```python
from build123d import *
from build123d.topology import SkipClean

# Parameters (mm, degrees)
ESQUISSE1_R             = 3.5
ESQUISSE1_R_2           = 8.5
BOSS_EXTRU_1_DEPTH      = 7
ESQUISSE2_R             = 23
ESQUISSE2_R_2           = 8.5
BOSS_EXTRU_2_DEPTH      = 7
ESQUISSE3_R             = 10
ESQUISSE3_R_2           = 8.5
BOSS_EXTRU_3_DEPTH      = 5.5
ENL_V_START             = -2
ESQUISSE4_R             = 21
ESQUISSE4_R_2           = 10
ENL_V_MAT_EXTRU_1_DEPTH = 2


with BuildPart() as part:
    # Esquisse1 → Boss.-Extru.1 (new body)
    with BuildSketch(Plane.XY):
        with BuildLine():
            Line((11.717444642, 19.791449948), (6, 35.5))
            ThreePointArc((6, 35.5), (0, 37.604686356), (-6, 35.5))
            Line((-6, 35.5), (-11.717444642, 19.791449948))
            ThreePointArc((-11.717444642, 19.791449948), (-23, 0), (-11.717444642, -19.791449948))
            Line((-11.717444642, -19.791449948), (-6, -35.5))
            ThreePointArc((-6, -35.5), (0, -37.604686356), (6, -35.5))
            Line((6, -35.5), (11.717444642, -19.791449948))
            ThreePointArc((11.717444642, -19.791449948), (23, 0), (11.717444642, 19.791449948))
        make_face()
        with Locations((0, 28)):
            Circle(ESQUISSE1_R, mode=Mode.SUBTRACT)
        Circle(ESQUISSE1_R_2, mode=Mode.SUBTRACT)
        with Locations(Location((0, -28, 0), (0, 0, 180))):
            Circle(ESQUISSE1_R, mode=Mode.SUBTRACT)
    extrude(amount=BOSS_EXTRU_1_DEPTH)

    # Esquisse2 → Boss.-Extru.2 (add)
    with BuildSketch(Plane.XY.offset(7)):
        with Locations(Location((0, 0, 0), (0, 0, 120.627475448))):
            Circle(ESQUISSE2_R)
        Circle(ESQUISSE2_R_2, mode=Mode.SUBTRACT)
    extrude(amount=BOSS_EXTRU_2_DEPTH)

    # Esquisse3 → Boss.-Extru.3 (add)
    with SkipClean():  # the faces are left unmerged after this step: merging them gives an invalid solid
        with BuildSketch(Plane.XY.offset(14)):
            Circle(ESQUISSE3_R)
            Circle(ESQUISSE3_R_2, mode=Mode.SUBTRACT)
        extrude(amount=BOSS_EXTRU_3_DEPTH)

    # Esquisse4 → Enlèv. mat.-Extru.1 (cut)
    with SkipClean():  # the faces are left unmerged after this step: merging them gives an invalid solid
        with BuildSketch(Plane.XY.offset(14).offset(ENL_V_START)):
            Circle(ESQUISSE4_R)
            Circle(ESQUISSE4_R_2, mode=Mode.SUBTRACT)
        extrude(amount=ENL_V_MAT_EXTRU_1_DEPTH, mode=Mode.SUBTRACT)


solid = part.part
```
Design review of the part built by this model. Coordinates are the model's own, in mm. A direction names the side the tool comes from. Coordinates: 2 decimals unless noted, no trailing zeros. Order: outer loops, then holes, each group sorted by start corner. A loop starts at its lowest first (then second) coordinate and runs counter-clockwise, first axis right, second up.
1) Take a section at C-C, the plane x = 0. Give the boundary of the cut face in (y, z), and give its area (3 significant figures).
2) Mouldability with a two-part tool opening along X and no side actions: class faces 1 (the flat face through (8.899, 27.536, 3.451)), 2 (the flat face through (9, 5, 12)), 3 (the flat face through (10.9, 18.2, 14)) as +X half, -X half, draft (parallel to the pull), parting line (faces both ways), or undercut.
3) Take a section at D-D, the plane y = 16. Give the boundary of the cut face in (x, z), and give its area (3 significant figures).
4) Wall thickness on line 1 along Y through (x, z) = (0, 2.5); line 2 along Y through (x, z) = (0, 12.6); line 3 along Y through (x, z) = (0, 10.25): over which ranges is each line inside the solid? List them lowest first.
5) Clearance check with flat-ended pins moving along their axes: pin 1 (2 mm diameter, centred on y = 15, z = 6.5, fed in from +X); pin 2 (2 mm diameter, centred on x = 10, z = 10, fed in from -Y); pin 3 (2 mm diameter, centred on x = 15, y = 4, fed in from +Z); pin 4 (5.5 mm diameter, centred on x = 0, y = 28, fed in from -Z). State where each tip first meets the part, or that it passes through.
6) Take a section at B-B, the plane z = 4.5. Give the boundary of the cut face in (x, y), and give its area (3 significant figures).
7) For faces 4 (the cylindrical face through (-2.17, -9.76, 15.7)), 5 (the cylindrical face through (-0.091, -37.604, 3.451)), list the 3-axis set-ups (+Z, -Z, +X, -X, +Y, -Y) from which the entire face can be reached by the end or side of a thin tool; tool diameter is ignored.
8) Take a section at A-A, the plane y = 0. Give the boundary of the cut face in (x, z), and give its area (4 significant figures).
Returned:
1. outline: (-37.6, 0) - (-31.5, 0) - (-31.5, 7) - (-37.6, 7) - close; (-24.5, 0) - (-8.5, 0) - (-8.5, 19.5) - (-10, 19.5) - (-10, 12) - (-21, 12) - (-21, 14) - (-23, 14) - (-23, 7) - (-24.5, 7) - close; (8.5, 0) - (24.5, 0) - (24.5, 7) - (23, 7) - (23, 14) - (21, 14) - (21, 12) - (10, 12) - (10, 19.5) - (8.5, 19.5) - close; (31.5, 0) - (37.6, 0) - (37.6, 7) - (31.5, 7) - close
1. area: 485 mm2
2. face 1: +X half
2. face 2: undercut
2. face 3: draft
3. outline: (-16.52, 0) - (16.52, 0) - (16.52, 14) - (13.6, 14) - (13.6, 12) - (-13.6, 12) - (-13.6, 14) - (-16.52, 14) - close
3. area: 408 mm2
4. line 1: y = -37.6 to -31.5, -24.5 to -8.5, 8.5 to 24.5, 31.5 to 37.6
4. line 2: y = -23 to -21, -10 to -8.5, 8.5 to 10, 21 to 23
4. line 3: y = -23 to -8.5, 8.5 to 23
5. pin 1: stops at x = 18.25
5. pin 2: stops at y = -21.17
5. pin 3: stops at z = 12
5. pin 4: passes through
6. outline: (-11.72, -19.79) - (-6, -35.5) arc R9.6 ccw to (6, -35.5) - (11.72, -19.79) arc R23 ccw to (11.72, 19.79) - (6, 35.5) arc R9.6 ccw to (-6, 35.5) - (-11.72, 19.79) arc R23 ccw to start; hole circle Ø17 at (0, 0); hole circle Ø7 at (0, -28); hole circle Ø7 at (0, 28)
6. area: 1,850 mm2
7. face 4: +Z
7. face 5: +Z, -Z, -Y
8. outline: (-23, 0) - (-8.5, 0) - (-8.5, 19.5) - (-10, 19.5) - (-10, 12) - (-21, 12) - (-21, 14) - (-23, 14) - close; (8.5, 0) - (23, 0) - (23, 14) - (21, 14) - (21, 12) - (10, 12) - (10, 19.5) - (8.5, 19.5) - close
8. area: 378.5 mm2
